from build123d import *

# Parameters (mm, degrees)
SKETCH_1_W                    = 210
SKETCH_1_H                    = 210
EXTRUDE_1_DEPTH               = 4
FILLET_1_SIZE                 = 20
HOLE_WIZARD_M31_D             = 3.15
HOLE_WIZARD_M31_DEPTH         = 8
HOLE_WIZARD_M31_TIP           = 0.946355475
HOLE_WIZARD_M35_D             = 3.4
HOLE_WIZARD_M35_CSINK_D       = 3.45
HOLE_WIZARD_M35_CSINK_ANGLE   = 90
HOLE_WIZARD_M31_2_D           = 3.2
HOLE_WIZARD_M31_2_DEPTH       = 4
HOLE_WIZARD_M31_2_CSINK_D     = 6.3
HOLE_WIZARD_M31_2_CSINK_ANGLE = 90
HOLE_WIZARD_M31_2_TIP         = 0.96137699
SKETCH_45_W                   = 71
SKETCH_45_H                   = 13
CUT_EXTRUDE_3_DEPTH           = 149.546289226
CUT_EXTRUDE_2_REACH           = 150.546
SKETCH_17_W                   = 28
SKETCH_17_H                   = 13.5
SKETCH_17_H_2                 = 4
FILLET_2_R                    = 2
FILLET_3_R                    = 3
FILLET_5_R                    = 3
HOLE_WIZARD_M32_D             = 3.4
HOLE_WIZARD_M32_CSINK_D       = 6.3
HOLE_WIZARD_M32_CSINK_ANGLE   = 90


with BuildPart() as part:
    # Эскиз1 → Бобышка-Вытянуть1 (new body)
    with BuildSketch(Plane(origin=(0, 0, 0), x_dir=(1, 0, 0), z_dir=(0, 1, 0))):
        Rectangle(SKETCH_1_W, SKETCH_1_H)
    extrude(amount=EXTRUDE_1_DEPTH)

    # Скругление1
    # a fillet whose section is not a circle: 20 mm, written as the material it takes off along each edge
    with BuildSketch(Plane(origin=(-105, -50, -105), x_dir=(1, 0, 0), z_dir=(0, 1, 0)), Plane(origin=(105, -50, -105), x_dir=(0, 0, 1), z_dir=(0, 1, 0)), Plane(origin=(105, -50, 105), x_dir=(-1, 0, 0), z_dir=(0, 1, 0))) as fillet_1_piece_1:
        with BuildLine():
            add(Edge.make_bspline([(FILLET_1_SIZE, 0), (FILLET_1_SIZE * 0.831801948466, 0), (FILLET_1_SIZE * 0.663603896932, 0), (FILLET_1_SIZE * 0.292893218813, -FILLET_1_SIZE * 0.0716919198361), (FILLET_1_SIZE * 0.0716919198361, -FILLET_1_SIZE * 0.292893218813), (0, -FILLET_1_SIZE * 0.663603896932), (0, -FILLET_1_SIZE * 0.831801948466), (0, -FILLET_1_SIZE)], knots=[0, 0, 0, 0, 0, 0, 0.5, 0.5, 1, 1, 1, 1, 1, 1], degree=5))
            Line((0, -FILLET_1_SIZE), (0, 0))
            Line((0, 0), (FILLET_1_SIZE, 0))
        make_face()
    extrude(amount=104, mode=Mode.SUBTRACT)
    with BuildSketch(Plane(origin=(-105, -50, 105), x_dir=(1, 0, 0), z_dir=(0, 1, 0))) as fillet_1_piece_2:
        with BuildLine():
            add(Edge.make_bspline([(FILLET_1_SIZE, 0), (FILLET_1_SIZE * 0.831801948466, 0), (FILLET_1_SIZE * 0.663603896932, 0), (FILLET_1_SIZE * 0.292893218813, FILLET_1_SIZE * 0.0716919198361), (FILLET_1_SIZE * 0.0716919198361, FILLET_1_SIZE * 0.292893218813), (0, FILLET_1_SIZE * 0.663603896932), (0, FILLET_1_SIZE * 0.831801948466), (0, FILLET_1_SIZE)], knots=[0, 0, 0, 0, 0, 0, 0.5, 0.5, 1, 1, 1, 1, 1, 1], degree=5))
            Line((0, FILLET_1_SIZE), (0, 0))
            Line((0, 0), (FILLET_1_SIZE, 0))
        make_face()
    extrude(amount=104, mode=Mode.SUBTRACT)

    # Hole Wizard M31
    with Locations(Plane(origin=(0, 4, 0), x_dir=(1, 0, 0), z_dir=(0, 1, 0))):
        with Locations((-68, 59.75), (-52, 59.75), (-68, 45.75), (-52, 45.75), (-52, -59.75), (-52, -45.75), (-68, -59.75), (52, -59.75), (52, -45.75), (68, -59.75), (68, -45.75), (52, 59.75), (52, 45.75), (-68, -45.75), (68, 45.75), (68, 59.75)):
            Hole(HOLE_WIZARD_M31_D / 2, depth=HOLE_WIZARD_M31_DEPTH)
            with Locations((0, 0, -(HOLE_WIZARD_M31_DEPTH + HOLE_WIZARD_M31_TIP / 2))):  # 118° drill point
                Cone(0, HOLE_WIZARD_M31_D / 2, HOLE_WIZARD_M31_TIP, mode=Mode.SUBTRACT)

    # Отверстие с зазором M35 (through all)
    with Locations(Plane(origin=(0, 4, 0), x_dir=(1, 0, 0), z_dir=(0, 1, 0))):
        with Locations((90, 66), (-90, 66), (-90, -66), (90, -66), (0, -90), (0, 90)):
            CounterSinkHole(HOLE_WIZARD_M35_D / 2, HOLE_WIZARD_M35_CSINK_D / 2, counter_sink_angle=HOLE_WIZARD_M35_CSINK_ANGLE)

    # Hole Wizard M31 2
    with Locations(Plane(origin=(0, 4, 0), x_dir=(1, 0, 0), z_dir=(0, 1, 0))):
        with Locations((28.2, 40), (-28.2, 40), (-28.2, -40), (28.2, -40)):
            CounterSinkHole(HOLE_WIZARD_M31_2_D / 2, HOLE_WIZARD_M31_2_CSINK_D / 2, depth=HOLE_WIZARD_M31_2_DEPTH, counter_sink_angle=HOLE_WIZARD_M31_2_CSINK_ANGLE)
            with Locations((0, 0, -(HOLE_WIZARD_M31_2_DEPTH + HOLE_WIZARD_M31_2_TIP / 2))):  # 118° drill point
                Cone(0, HOLE_WIZARD_M31_2_D / 2, HOLE_WIZARD_M31_2_TIP, mode=Mode.SUBTRACT)

    # Эскиз45 → Вырез-Вытянуть3 (cut, through all)
    with BuildSketch(Plane(origin=(0, 4, 0), x_dir=(1, 0, 0), z_dir=(0, 1, 0))):
        with Locations((-60, 90)):
            Rectangle(SKETCH_45_W, SKETCH_45_H)
        with Locations((-60, -90)):
            Rectangle(SKETCH_45_W, SKETCH_45_H)
        with Locations((60, -90)):
            Rectangle(SKETCH_45_W, SKETCH_45_H)
        with Locations((60, 90)):
            Rectangle(SKETCH_45_W, SKETCH_45_H)
    extrude(amount=-CUT_EXTRUDE_3_DEPTH, mode=Mode.SUBTRACT)

    # Эскиз17 → Вырез-Вытянуть2 (cut, up to next)
    with BuildSketch(Plane(origin=(0, 4, 0), x_dir=(1, 0, 0), z_dir=(0, 1, 0)), mode=Mode.PRIVATE) as cut_extrude_2_sk1:
        with Locations((-60, 76.75)):
            Rectangle(SKETCH_17_W, SKETCH_17_H)
    cut_extrude_2_tool1 = extrude(cut_extrude_2_sk1.sketch, amount=-CUT_EXTRUDE_2_REACH, mode=Mode.PRIVATE) & part.part
    # Эскиз17 → Вырез-Вытянуть2 (cut, up to next)
    with BuildSketch(Plane(origin=(0, 4, 0), x_dir=(1, 0, 0), z_dir=(0, 1, 0)), mode=Mode.PRIVATE) as cut_extrude_2_sk2:
        with Locations((-60, 68)):
            Rectangle(SKETCH_17_W, SKETCH_17_H_2)
    cut_extrude_2_tool2 = extrude(cut_extrude_2_sk2.sketch, amount=-CUT_EXTRUDE_2_REACH, mode=Mode.PRIVATE) & part.part
    # Эскиз17 → Вырез-Вытянуть2 (cut, up to next)
    with BuildSketch(Plane(origin=(0, 4, 0), x_dir=(1, 0, 0), z_dir=(0, 1, 0)), mode=Mode.PRIVATE) as cut_extrude_2_sk3:
        Polygon((-46, -70), (-46, -83.5), (-74, -83.5), (-74, -70), (-74, -66), (-46, -66), align=None)
    cut_extrude_2_tool3 = extrude(cut_extrude_2_sk3.sketch, amount=-CUT_EXTRUDE_2_REACH, mode=Mode.PRIVATE) & part.part
    # Эскиз17 → Вырез-Вытянуть2 (cut, up to next)
    with BuildSketch(Plane(origin=(0, 4, 0), x_dir=(1, 0, 0), z_dir=(0, 1, 0)), mode=Mode.PRIVATE) as cut_extrude_2_sk4:
        Polygon((74, -83.5), (46, -83.5), (46, -70), (46, -66), (74, -66), (74, -70), align=None)
    cut_extrude_2_tool4 = extrude(cut_extrude_2_sk4.sketch, amount=-CUT_EXTRUDE_2_REACH, mode=Mode.PRIVATE) & part.part
    # Эскиз17 → Вырез-Вытянуть2 (cut, up to next)
    with BuildSketch(Plane(origin=(0, 4, 0), x_dir=(1, 0, 0), z_dir=(0, 1, 0)), mode=Mode.PRIVATE) as cut_extrude_2_sk5:
        Polygon((46, 70), (46, 83.5), (74, 83.5), (74, 70), (74, 66), (46, 66), align=None)
    cut_extrude_2_tool5 = extrude(cut_extrude_2_sk5.sketch, amount=-CUT_EXTRUDE_2_REACH, mode=Mode.PRIVATE) & part.part
    add(cut_extrude_2_tool1.solids().sort_by_distance((-60, 4, -76.75))[0], mode=Mode.SUBTRACT)
    add(cut_extrude_2_tool2.solids().sort_by_distance((-60, 4, -68))[0], mode=Mode.SUBTRACT)
    add(cut_extrude_2_tool3.solids().sort_by_distance((-60, 4, 74.75))[0], mode=Mode.SUBTRACT)
    add(cut_extrude_2_tool4.solids().sort_by_distance((60, 4, 74.75))[0], mode=Mode.SUBTRACT)
    add(cut_extrude_2_tool5.solids().sort_by_distance((60, 4, -74.75))[0], mode=Mode.SUBTRACT)

    # Скругление2
    fillet_2_edges = [part.edges().sort_by_distance(p)[0] for p in [
        (46, 2, 66),
        (74, 2, 66),
        (-46, 2, 66),
        (-74, 2, 66),
        (-74, 2, -66),
        (-46, 2, -66),
    ]]
    fillet(fillet_2_edges, radius=FILLET_2_R)

    # Скругление3
    fillet_3_edges = [part.edges().sort_by_distance(p)[0] for p in [
        (46, 2, -83.5),
        (74, 2, -83.5),
        (74, 2, 83.5),
        (46, 2, 83.5),
        (-46, 2, 83.5),
        (-74, 2, 83.5),
        (-74, 2, -83.5),
        (-46, 2, -83.5),
    ]]
    fillet(fillet_3_edges, radius=FILLET_3_R)

    # Скругление5
    fillet_5_edges = [part.edges().sort_by_distance(p)[0] for p in [
        (-95.5, 2, 83.5),
        (-24.5, 2, 83.5),
        (-24.5, 2, 96.5),
        (-95.5, 2, 96.5),
        (95.5, 2, 96.5),
        (24.5, 2, 96.5),
        (24.5, 2, 83.5),
        (95.5, 2, 83.5),
        (95.5, 2, -83.5),
        (24.5, 2, -83.5),
        (24.5, 2, -96.5),
        (95.5, 2, -96.5),
        (-24.5, 2, -96.5),
        (-24.5, 2, -83.5),
        (-95.5, 2, -83.5),
        (-95.5, 2, -96.5),
    ]]
    fillet(fillet_5_edges, radius=FILLET_5_R)

    # Зенковка для винта с полупотайной головкой M32 (through all)
    with Locations(Plane(origin=(0, 0, 0), x_dir=(-1, 0, 0), z_dir=(0, -1, 0))):
        with Locations((39.01939717, 19.466602706), (6.98060283, 19.466602706), (6.98060283, -19.466602706), (39.01939717, -19.466602706)):
            CounterSinkHole(HOLE_WIZARD_M32_D / 2, HOLE_WIZARD_M32_CSINK_D / 2, counter_sink_angle=HOLE_WIZARD_M32_CSINK_ANGLE)


solid = part.part
Verification items for the finished model (mm, model axes). Coordinates: 2 decimals unless noted, no trailing zeros. Order: outer loops, then holes, each group sorted by start corner. A loop starts at its lowest first (then second) coordinate and runs counter-clockwise, first axis right, second up. Notation, with made-up numbers: M 35.25,-37.5 L 88.25,-37.5 A28 cw 88.25,-10.5 Z; hole C -28.5,29.5 d10. An arc over 180 degrees is marked long. One line per item, written item: value. Start each with the question number.
Item 1: Sectioned sample at A-A on x = 59.5. Record the cut outline in (y, z).
Item 2: Sectioned sample at B-B on z = -73.5. Record the cut outline in (x, y), then the cut area to 3 significant figures.
Item 3: Thickness scan on probe 1 along Z at (x, y) = (-39, 2.95); probe 2 along Z at (x, y) = (-85.5, 0.8); probe 3 along X at (y, z) = (2.3, 59.75) (3 decimals). Record the ranges inside material, lowest first.
Item 4: Depth check by flat-ended pin: P1, Ø1.2, axis at y = 2.5, z = 91.5, coming from the -X side; P2, Ø1.9, axis at x = 52, z = -59.75, coming from the -Y side; P3, Ø2, axis at y = 2.5, z = -91.5, coming from the +X side; P4, Ø2, axis at y = 2, z = 90, coming from the +X side. Enter the tip coordinate at first touch or a pass-through.
Calculated:
1. outline: M 0,-105 L 4,-105 L 4,-96.5 L 0,-96.5 Z; M 0,-66 L 4,-66 L 4,66 L 0,66 Z; M 0,96.5 L 4,96.5 L 4,105 L 0,105 Z
2. outline: M -105,0 L -74,0 L -74,4 L -105,4 Z; M -46,0 L 46,0 L 46,4 L -46,4 Z; M 74,0 L 105,0 L 105,4 L 74,4 Z
2. area: 616 mm^2
3. probe 1: -105 to -96.5, -83.5 to -21.17, -17.77 to 17.77, 21.17 to 83.5, 96.5 to 105
3. probe 2: -105 to -96.5, -83.5 to 83.5, 96.5 to 105
3. probe 3: -105 to -69.575, -66.425 to -53.575, -50.425 to 50.425, 53.575 to 66.425, 69.575 to 105
4. P1: x = -104.75
4. P2: through
4. P3: x = 104.79
4. P4: x = 104.92
